Here's the drawing with two shaded views (mm, measured from the low corner). I have some questions. A direction names the side the tool comes from. Round coordinates to 2 decimals unless told otherwise and drop trailing zeros. Order: outer loops, then holes, each group sorted by start corner. A loop starts at its lowest first (then second) coordinate and runs counter-clockwise, first axis right, second up. Notation, with made-up numbers: (46.25, -6.75) -> (89.25, -6.75) arc R15 ccw to (89.25, 6.25) -> close; hole circle Ø7 at (88, 52.5). An arc over 180 degrees is marked (long way). Answer in a Markdown table with one row per item.
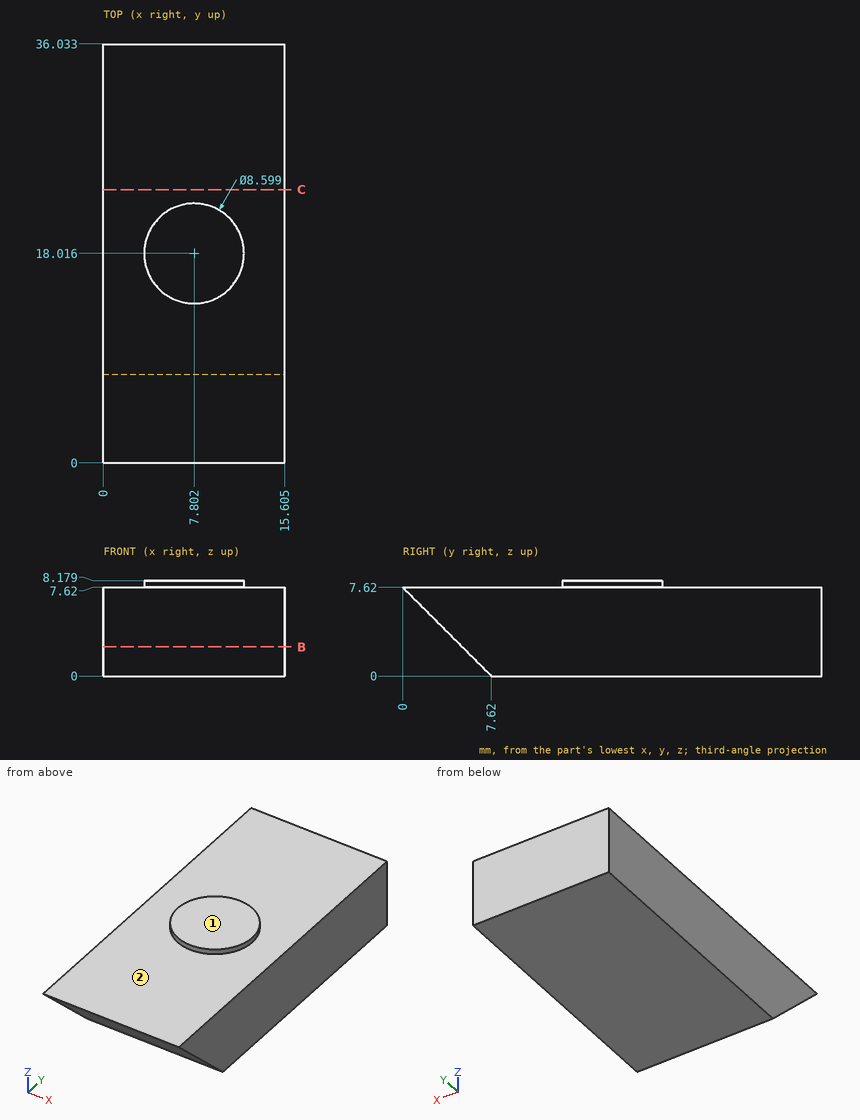
1. For pin 1 Ø2 at (x, z) = (10, 6) entering from -Y, with a flat end and sliding along its axis, tell me the tip position at first contact or that it passes through.
Numbers:
| item | result |
|---|---|
| pin 1 | stops at y = 0.62 |
2. For the marked faces 1 and 2, which set-ups out of +Z, -Z, +X, -X, +Y, -Y let a thin tool reach every point of the face, with its end or its side?
Numbers:
| item | result |
|---|---|
| face 1 | +Z, +X, -X, +Y, -Y |
| face 2 | +Z |
3. Suppose I cut it at C-C on y = 23.5. Write out the boundary of the cut face in (x, z) (1 decimal).
Numbers:
| item | result |
|---|---|
| outline | (0, 0) -> (15.6, 0) -> (15.6, 7.6) -> (0, 7.6) -> close |
4. Please list where these lines run through material, in increasing order: line 1 along Z through (x, y) = (2, 33.5); line 2 along Z through (x, y) = (3.5, 2.5); line 3 along Y through (x, z) = (7.25, 4) (1 decimal).
Numbers:
| item | result |
|---|---|
| line 1 | z = 0 to 7.62 |
| line 2 | z = 5.12 to 7.62 |
| line 3 | y = 3.6 to 36 |
5. Suppose I cut it at B-B on z = 2.5. Write out the boundary of the cut face in (x, y) (1 decimal).
Numbers:
| item | result |
|---|---|
| outline | (0, 5.1) -> (15.6, 5.1) -> (15.6, 36) -> (0, 36) -> close |
